Geometry: final body of the model. Coordinates: model frame, mm. Face numbers are marked on the shaded views. A direction names the side the tool comes from. Give positions to 0.01 mm unless a question says otherwise; leave off trailing zeros. Loops run counter-clockwise (first coordinate to the right, second up) from the corner with the lowest first, then second, coordinate; pieces in that order, holes last.
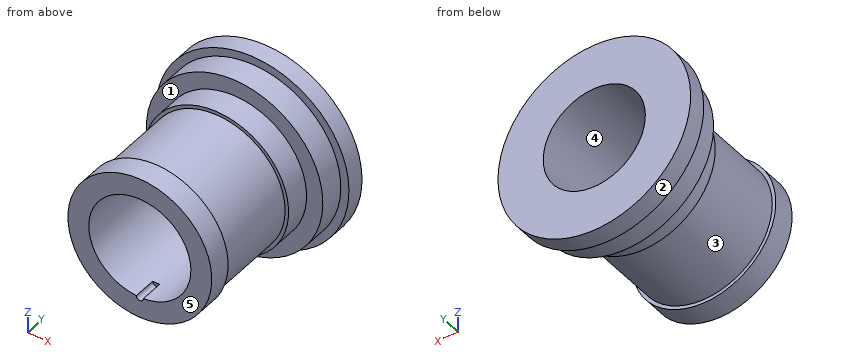
from build123d import *

# Parameters (mm, degrees)
SKETCH4_R          = 22
CUT_EXTRUDE1_DEPTH = 78
SKETCH5_R          = 1.5
CUT_EXTRUDE2_DEPTH = 10


with BuildPart() as part:
    # Sketch3 → Revolve1 (revolve)
    with BuildSketch(Plane.XY, mode=Mode.PRIVATE) as revolve1_sk:
        Polygon((0, 0), (31, 0), (31, 10), (29.5, 10), (29.5, 47), (31, 47), (31, 58), (38, 58), (38, 69), (41.5, 69), (41.5, 77), (0, 77), align=None)
    revolve(revolve1_sk.sketch.rotate(Axis((0, 98.317518248, 0), (0, -1, 0)), 90), axis=Axis((0, 98.317518248, 0), (0, -1, 0)))  # turned: the seam where the file's is

    # Sketch4 → Cut-Extrude1 (cut, through all)
    with BuildSketch(Plane(origin=(0, 77, 0), x_dir=(1, 0, 0), z_dir=(0, 1, 0))):
        with Locations(Location((0, 0, 0), (0, 0, 270))):  # turned: the seam where the file's is
            Circle(SKETCH4_R)
    extrude(amount=-CUT_EXTRUDE1_DEPTH, mode=Mode.SUBTRACT)

    # Sketch5 → Cut-Extrude2 (cut)
    with BuildSketch(Plane(origin=(0, 0, 0), x_dir=(-1, 0, 0), z_dir=(0, -1, 0))):
        with Locations((0, 22)):
            Circle(SKETCH5_R)
    extrude(amount=-CUT_EXTRUDE2_DEPTH, mode=Mode.SUBTRACT)


solid = part.part
Item 1: Draft query along X for the marked faces 3, 4 and 5. Return one class per face: +X half, -X half, draft (parallel to the pull), parting line (faces both ways), or undercut.
Values follow:
face 3: parting line
face 4: undercut
face 5: draft
Item 2: Section query D-D on z = -13.5. Return loops of the section in (x, y).
Values follow:
outline: (-39.24, 69) - (-35.52, 69) - (-35.52, 58) - (-27.91, 58) - (-27.91, 47) - (-26.23, 47) - (-26.23, 10) - (-27.91, 10) - (-27.91, 0) - (-17.37, 0) - (-17.37, 77) - (-39.24, 77) - close; (17.37, 0) - (27.91, 0) - (27.91, 10) - (26.23, 10) - (26.23, 47) - (27.91, 47) - (27.91, 58) - (35.52, 58) - (35.52, 69) - (39.24, 69) - (39.24, 77) - (17.37, 77) - close
Item 3: Section query A-A on x = 0. Return loops of the section in (y, z).
Values follow:
outline: (0, -31) - (10, -31) - (10, -29.5) - (47, -29.5) - (47, -31) - (58, -31) - (58, -38) - (69, -38) - (69, -41.5) - (77, -41.5) - (77, -22) - (10, -22) - (10, -23.5) - (0, -23.5) - close; (0, 22) - (77, 22) - (77, 41.5) - (69, 41.5) - (69, 38) - (58, 38) - (58, 31) - (47, 31) - (47, 29.5) - (10, 29.5) - (10, 31) - (0, 31) - close
Item 4: Set-up query: the marked faces 1 and 2. Return all of +Z, -Z, +X, -X, +Y, -Y with unobstructed straight access to the full face (end or side cutting, diameter ignored); none if empty.
Values follow:
face 1: -Y
face 2: +Y, -Y
Item 5: Pin query (flat end, axial travel): pin 1 (18.5 mm diameter, centred on x = -10, z = 0, fed in from +Y); pin 2 (10 mm diameter, centred on y = 67.5, z = -30.5, fed in from -X); pin 3 (0.5 mm diameter, centred on x = -0.5, z = -22.5, fed in from -Y); pin 4 (4 mm diameter, centred on y = 37.5, z = -27, fed in from -X). Return the tip coordinate at first contact, or that it passes through.
Values follow:
pin 1: passes through
pin 2: stops at x = -32.56
pin 3: stops at y = 10
pin 4: stops at x = -15.66
Item 6: Section query C-C on y = 44.5. Return loops of the section in (x, z).
Values follow:
outline: circle Ø59 at (0, 0); hole circle Ø44 at (0, 0)
Item 7: Section query B-B on z = 0. Return loops of the section in (x, y), plus the area to 3 significant figures.
Values follow:
outline: (-41.5, 69) - (-38, 69) - (-38, 58) - (-31, 58) - (-31, 47) - (-29.5, 47) - (-29.5, 10) - (-31, 10) - (-31, 0) - (-22, 0) - (-22, 77) - (-41.5, 77) - close; (22, 0) - (31, 0) - (31, 10) - (29.5, 10) - (29.5, 47) - (31, 47) - (31, 58) - (38, 58) - (38, 69) - (41.5, 69) - (41.5, 77) - (22, 77) - close
area: 1,600 mm2
Item 8: Ray query, probe 1 along Y at (x, z) = (2.5, 30); probe 2 along X at (y, z) = (45.5, 0); probe 3 along Y at (x, z) = (33, 4). Return the intervals inside material, ascending.
Values follow:
probe 1: y = 0 to 10, 47 to 77
probe 2: x = -29.5 to -22, 22 to 29.5
probe 3: y = 58 to 77
